Geometry: final body of the model. Coordinates: model frame, mm. A direction names the side the tool comes from. Give positions to 0.01 mm unless a question says otherwise; leave off trailing zeros. Order: outer loops, then holes, each group sorted by start corner. A loop starts at its lowest first (then second) coordinate and runs counter-clockwise, first axis right, second up. Notation, with made-up numbers: (-37.5, 19.25) -> (-30.5, 19.25) arc R20 cw to (-30.5, 42.25) -> close; hole circle Ø3 at (10.5, 32.5). An arc over 180 degrees is marked (long way). One line per question, with ' | ' between items.
from build123d import *

# Parameters (mm, degrees)
SKETCH1_W                          = 12
SKETCH1_H                          = 12
BOSS_EXTRUDE1_DEPTH                = 11.5
SKETCH2_W                          = 12
SKETCH2_H                          = 12
SKETCH2_W_2                        = 10
SKETCH2_H_2                        = 10
BOSS_EXTRUDE2_DEPTH                = 1
F_1_0MM_DOWEL_HOLE1_D              = 1
F_1_0MM_DOWEL_HOLE1_DEPTH          = 1
F_1_16_0_0625_DIAMETER_HOLE1_D     = 1.5875
F_1_16_0_0625_DIAMETER_HOLE1_DEPTH = 7.5
M2X0_4_TAPPED_HOLE1_D              = 1.6
M2X0_4_TAPPED_HOLE1_DEPTH          = 5.2
M2X0_4_TAPPED_HOLE1_TIP            = 0.480688495


with BuildPart() as part:
    # Sketch1 → Boss-Extrude1 (new body)
    with BuildSketch(Plane(origin=(0, 0, 0), x_dir=(1, 0, 0), z_dir=(0, 1, 0))):
        Rectangle(SKETCH1_W, SKETCH1_H)
    extrude(amount=BOSS_EXTRUDE1_DEPTH)

    # Sketch2 → Boss-Extrude2 (add)
    with BuildSketch(Plane(origin=(0, 11.5, 0), x_dir=(1, 0, 0), z_dir=(0, 1, 0))):
        Rectangle(SKETCH2_W, SKETCH2_H)
        Rectangle(SKETCH2_W_2, SKETCH2_H_2, mode=Mode.SUBTRACT)
    extrude(amount=BOSS_EXTRUDE2_DEPTH)

    # Ø1.0mm Dowel Hole1
    with Locations(Plane(origin=(0, 12.5, 0), x_dir=(1, 0, 0), z_dir=(0, 1, 0))):
        with Locations((-5, 5), (5, 5), (5, -5), (-5, -5)):
            Hole(F_1_0MM_DOWEL_HOLE1_D / 2, depth=F_1_0MM_DOWEL_HOLE1_DEPTH)

    # 1/16 (0.0625) Diameter Hole1
    with Locations(Plane(origin=(0, 0, 0), x_dir=(-1, 0, 0), z_dir=(0, -1, 0))):
        with Locations((3.878679656, 3.878679656), (-3.878679656, -3.878679656)):
            Hole(F_1_16_0_0625_DIAMETER_HOLE1_D / 2, depth=F_1_16_0_0625_DIAMETER_HOLE1_DEPTH)

    # M2x0.4 Tapped Hole1
    with Locations(Plane(origin=(0, 0, 0), x_dir=(-1, 0, 0), z_dir=(0, -1, 0))):
        with Locations((3.878679656, -3.878679656), (-3.878679656, 3.878679656)):
            Hole(M2X0_4_TAPPED_HOLE1_D / 2, depth=M2X0_4_TAPPED_HOLE1_DEPTH)
            with Locations((0, 0, -(M2X0_4_TAPPED_HOLE1_DEPTH + M2X0_4_TAPPED_HOLE1_TIP / 2))):  # 118° drill point
                Cone(0, M2X0_4_TAPPED_HOLE1_D / 2, M2X0_4_TAPPED_HOLE1_TIP, mode=Mode.SUBTRACT)


solid = part.part
1) Section B-B on y = 4. Return loops of the section in (x, z), plus the area to 3 significant figures.
Check result:
outline: (-6, -6) -> (6, -6) -> (6, 6) -> (-6, 6) -> close; hole circle Ø1.6 at (-3.88, 3.88); hole circle Ø1.59 at (-3.88, -3.88); hole circle Ø1.6 at (3.88, -3.88); hole circle Ø1.59 at (3.88, 3.88) | area: 136 mm^2
2) Section A-A on z = -2.75. Return loops of the section in (x, y), plus the area to 3 significant figures.
Check result:
outline: (-6, 0) -> (6, 0) -> (6, 12.5) -> (5, 12.5) -> (5, 11.5) -> (-5, 11.5) -> (-5, 12.5) -> (-6, 12.5) -> close | area: 140 mm^2
3) Material intervals for probe 1 along X at (y, z) = (3.25, 4); probe 2 along Z at (x, y) = (4.25, 4.75); probe 3 along X at (y, z) = (12.25, 1.25), sorted ascending. Write a range as from..to.
Check result:
probe 1: x = -6..-4.67, -3.09..3.09, 4.66..6 | probe 2: z = -6..-4.59, -3.17..3.18, 4.58..6 | probe 3: x = -6..-5, 5..6
4) Contact query for flat-ended pins moving along their axis: pin 1 Ø1 at (x, z) = (3.88, 3.88) entering from -Y; pin 2 Ø1 at (x, z) = (-3.88, 3.88) entering from -Y; pin 3 Ø3.5 at (x, z) = (-2, 0.5) entering from +Y. Output: stop coordinate, or through.
Check result:
pin 1: stops at y = 7.5 | pin 2: stops at y = 5.38 | pin 3: stops at y = 11.5
5) Set-up query: faces 4 (the cylindrical face through (-3.116, 2.636, 3.638)), 5 (the flat face through (0, 11.5, 0)), 6 (the flat face through (-6, 6, 0)). Return all of +Z, -Z, +X, -X, +Y, -Y with unobstructed straight access to the full face (end or side cutting, diameter ignored); none if empty.
Check result:
face 4: -Y | face 5: +Y | face 6: +Z, -Z, -X, +Y, -Y
6) Section C-C on x = -1.5. Return loops of the section in (y, z), plus the area to 3 significant figures.
Check result:
outline: (0, -6) -> (12.5, -6) -> (12.5, -5) -> (11.5, -5) -> (11.5, 5) -> (12.5, 5) -> (12.5, 6) -> (0, 6) -> close | area: 140 mm^2
7) Pull-direction query (Z, two-part tool) for faces 1 (the flat face through (0, 6, -6)), 2 (the cylindrical face through (-5.4, 12, -5.3)), 3 (the flat face through (6, 6, 0)); classes: +Z half, -Z half, draft (parallel to the pull), parting line (faces both ways), or undercut.
Check result:
face 1: -Z half | face 2: undercut | face 3: draft
